The model under review builds one solid part; all positions refer to its coordinate system, in mm. Round coordinates to 2 decimals unless told otherwise and drop trailing zeros. Order: outer loops, then holes, each group sorted by start corner. A loop starts at its lowest first (then second) coordinate and runs counter-clockwise, first axis right, second up.
```python
from build123d import *

# Parameters (mm, degrees)
SKETCH1_W           = 1143
SKETCH1_H           = 508
BOSS_EXTRUDE1_DEPTH = 6.35
CUT_EXTRUDE1_DEPTH  = 7.35
CUT_EXTRUDE2_DEPTH  = 7.35


with BuildPart() as part:
    # Sketch1 → Boss-Extrude1 (new body)
    with BuildSketch(Plane.XY):
        with Locations((571.5, 254)):
            Rectangle(SKETCH1_W, SKETCH1_H)
    extrude(amount=BOSS_EXTRUDE1_DEPTH)

    # Sketch2 → Cut-Extrude1 (cut, through all)
    with BuildSketch(Plane.XY.offset(6.35)):
        with BuildLine():
            Line((431.8, 450.85), (495.3, 450.85))
            ThreePointArc((495.3, 450.85), (511.175, 434.975), (495.3, 419.1))
            Line((495.3, 419.1), (431.8, 419.1))
            ThreePointArc((431.8, 419.1), (415.925, 434.975), (431.8, 450.85))
        make_face()
        with BuildLine():
            Line((685.8, 450.85), (749.3, 450.85))
            ThreePointArc((749.3, 450.85), (765.175, 434.975), (749.3, 419.1))
            Line((749.3, 419.1), (685.8, 419.1))
            ThreePointArc((685.8, 419.1), (669.925, 434.975), (685.8, 450.85))
        make_face()
    extrude(amount=-CUT_EXTRUDE1_DEPTH, mode=Mode.SUBTRACT)

    # Sketch6 → Cut-Extrude2 (cut, through all)
    with BuildSketch(Plane.XY.offset(6.35)):
        with BuildLine():
            Line((1038.225, 508), (1076.325, 508))
            Line((1076.325, 508), (1076.325, 495.3))
            ThreePointArc((1076.325, 495.3), (1057.275, 476.25), (1038.225, 495.3))
            Line((1038.225, 495.3), (1038.225, 508))
        make_face()
    extrude(amount=-CUT_EXTRUDE2_DEPTH, mode=Mode.SUBTRACT)


solid = part.part
```
(1) Consider section A-A (x = 696.5). Write out the cut boundary in (y, z), and give its area (3 significant figures).
Data:
outline: (0, 0) - (419.1, 0) - (419.1, 6.35) - (0, 6.35) - close; (450.85, 0) - (508, 0) - (508, 6.35) - (450.85, 6.35) - close
area: 3,020 mm2
(2) To check wall thickness, follow probe 1 along Y at (x, z) = (429.5, 3.5); probe 2 along X at (y, z) = (429, 2.75); probe 3 along Y at (x, z) = (676.5, 4.75). State the ranges of each line that lie inside material, in increasing order.
Data:
probe 1: y = 0 to 419.27, 450.68 to 508
probe 2: x = 0 to 417.09, 510.01 to 671.09, 764.01 to 1143
probe 3: y = 0 to 422.11, 447.84 to 508
(3) Draft analysis for pull direction X (two halves, no side actions). For faces 1 (the flat face through (563, 258, 6.35)), 2 (the cylindrical face through (1057.694, 476.255, 3.219)), state which applies: pulls with the +X half, pulls with the -X half, needs draft (parallel to the pull), parting line crosses it, or undercut.
Data:
face 1: needs draft
face 2: undercut
